Can you work these out from the model? Positions are in its coordinate system, mm. Face numbers are marked on the shaded views. A direction names the side the tool comes from. Coordinates: 2 decimals unless noted, no trailing zeros. Order: outer loops, then holes, each group sorted by start corner. A loop starts at its lowest first (then second) coordinate and runs counter-clockwise, first axis right, second up. Notation, with made-up numbers: M -23,18 L -4,18 A20 cw -4,23 Z; hole C 23.25,-38.5 d5. An arc over 180 degrees is marked long. Answer as a JSON object with one key per item and string values.
from build123d import *

# Parameters (mm, degrees)
SKETCH1_W                       = 94
SKETCH1_H                       = 170
BOSS_EXTRUDE1_DEPTH             = 10
CBORE_FOR_M5_SBHCS1_D           = 5.5
CBORE_FOR_M5_SBHCS1_CBORE_D     = 10.5
CBORE_FOR_M5_SBHCS1_CBORE_DEPTH = 3
SKETCH4_W                       = 94
SKETCH4_H                       = 60
BOSS_EXTRUDE2_DEPTH             = 8
FILLET1_R                       = 2
M4X0_7_TAPPED_HOLE1_D           = 3.3
M4X0_7_TAPPED_HOLE1_DEPTH       = 8


with BuildPart() as part:
    # Sketch1 → Boss-Extrude1 (new body)
    with BuildSketch(Plane.XY):
        with Locations((47, 85)):
            Rectangle(SKETCH1_W, SKETCH1_H)
    extrude(amount=BOSS_EXTRUDE1_DEPTH)

    # CBORE for M5 SBHCS1 (through all)
    with Locations(Plane.XY.offset(10)):
        with Locations((81.5, 157.5), (12.5, 85), (12.5, 157.5), (81.5, 85), (12.5, 12.5), (81.5, 12.5)):
            CounterBoreHole(CBORE_FOR_M5_SBHCS1_D / 2, CBORE_FOR_M5_SBHCS1_CBORE_D / 2, CBORE_FOR_M5_SBHCS1_CBORE_DEPTH)

    # Sketch4 → Boss-Extrude2 (add)
    with BuildSketch(Plane(origin=(0, 170, 0), x_dir=(1, 0, 0), z_dir=(0, 1, 0))):
        with Locations((47, 20)):
            Rectangle(SKETCH4_W, SKETCH4_H)
    extrude(amount=BOSS_EXTRUDE2_DEPTH)

    # Fillet1
    fillet1_edges = [part.edges().sort_by_distance(p)[0] for p in [
        (94, 89, 10),
        (0, 89, 10),
        (0, 174, -50),
        (94, 174, -50),
        (0, 178, -20),
        (47, 178, 10),
        (94, 178, -20),
        (47, 178, -50),
        (94, 0, 5),
        (0, 0, 5),
        (47, 0, 10),
    ]]
    fillet(fillet1_edges, radius=FILLET1_R)

    # M4x0.7 Tapped Hole1
    with Locations(Plane(origin=(0, 0, 0), x_dir=(-1, 0, 0), z_dir=(0, 0, -1))):
        with Locations((-47, 140), (-47, 49)):
            Hole(M4X0_7_TAPPED_HOLE1_D / 2, depth=M4X0_7_TAPPED_HOLE1_DEPTH)


solid = part.part
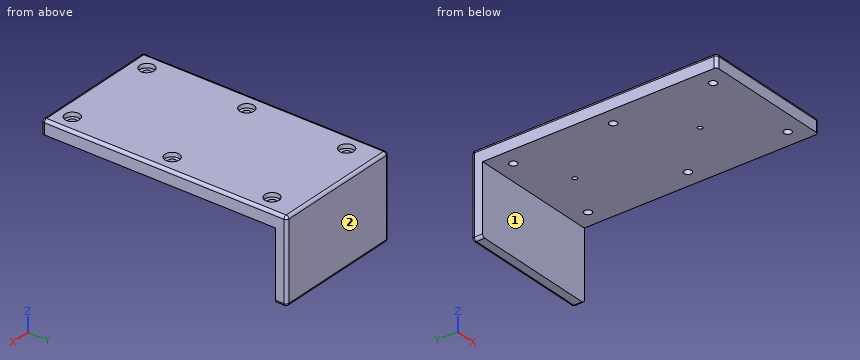
Item 1: I want a section at D-D, the plane z = -28. Write out the boundary of the cut face in (x, y), plus the area to 3 significant figures.
Answers follow:
{"outline": "M 0,170 L 94,170 L 94,176 A2 ccw 92,178 L 2,178 A2 ccw 0,176 Z", "area": "750 mm^2"}
Item 2: I want a section at C-C, the plane x = 58. Write out the boundary of the cut face in (y, z), plus the area to 3 significant figures.
Answers follow:
{"outline": "M 0,0 L 170,0 L 170,-50 L 176,-50 A2 ccw 178,-48 L 178,8 A2 ccw 176,10 L 2,10 A2 ccw 0,8 Z", "area": "2,180 mm^2"}
Item 3: I want a section at B-B, the plane x = 81.5. Give the number of separate pieces and of enclosed holes in the cut face, plus the area to 3 significant figures.
Answers follow:
{"separate pieces": "4", "enclosed holes": "0", "area": "1,970 mm^2"}
Item 4: Which directions (+Z, -Z, +X, -X, +Y, -Y) give clear straight access to the entire face, cutting with the end or side of a thin tool? Please do the marked faces 1 and 2.
Answers follow:
{"face 1": "-Z, +X, -X, -Y", "face 2": "+Z, -Z, +X, -X, +Y"}
Item 5: I'm going to push flat-ended pins straight in: pin 1 (7 mm diameter, centred on x = 81.5, y = 157.5, fed in from -Z); pin 2 (15 mm diameter, centred on x = 61.5, z = -15, fed in from -Y); pin 3 (5 mm diameter, centred on x = 82, y = 157, fed in from +Z). Where does each tip first touch, or does it pass through?
Answers follow:
{"pin 1": "stops at z = 0", "pin 2": "stops at y = 170", "pin 3": "stops at z = 7"}
Item 6: I want a section at A-A, the plane y = 12.5. Write out the boundary of the cut face in (x, z).
Answers follow:
{"outline": "M 0,0 L 9.75,0 L 9.75,7 L 7.25,7 L 7.25,10 L 2,10 A2 ccw 0,8 Z; M 15.25,0 L 78.75,0 L 78.75,7 L 76.25,7 L 76.25,10 L 17.75,10 L 17.75,7 L 15.25,7 Z; M 84.25,0 L 94,0 L 94,8 A2 ccw 92,10 L 86.75,10 L 86.75,7 L 84.25,7 Z"}
Item 7: Please list where these lines run through material, in increasing order: line 1 (Y direction, x = 12.5, z = 7.95); line 2 (Y direction, x = 47, z = 5); line 3 (X direction, y = 157.5, z = 5.25).
Answers follow:
{"line 1": "y = 0 to 7.25, 17.75 to 79.75, 90.25 to 152.25, 162.75 to 178", "line 2": "y = 0 to 47.35, 50.65 to 138.35, 141.65 to 178", "line 3": "x = 0 to 9.75, 15.25 to 78.75, 84.25 to 94"}
